Part model, mm, in its own coordinate system. A direction names the side the tool comes from. Round coordinates to 2 decimals unless told otherwise and drop trailing zeros. Order: outer loops, then holes, each group sorted by start corner. A loop starts at its lowest first (then second) coordinate and runs counter-clockwise, first axis right, second up. Notation, with made-up numbers: (-11, 46) -> (40, 46) arc R34 cw to (40, 79) -> close; hole circle Ø4 at (53, 10). An arc over 180 degrees is marked (long way). Return JSON: item names as keys, results as strings. Group by question number.
Autodesk Inventor part; units mm, degrees
ref_plane "YZ Plane" through (0, 0, 0) normal (1, 0, 0) x (0, 1, 0)
ref_plane "XZ Plane" through (0, 0, 0) normal (0, 1, 0) x (-1, 0, 0)
ref_plane "XY Plane" through (0, 0, 0) normal (0, 0, 1) x (1, 0, 0)
sketch "Sketch1" plane through (0, 0, 0) normal (0, 0, 1) x (1, 0, 0)
  circle A0 centre (0, 0) radius 14.75
  circle A1 centre (0, 0) radius 8 construction
  line L0 (-14.75, 0) -> (14.75, 0) construction
  line L1 (-7.5993, -2.5) -> (7.5993, -2.5) construction
  line L2 (-7.5993, 2.5) -> (7.5993, 2.5) construction
  circle A2 centre (0, 0) radius 12.5 construction
  circle A3 centre (0, 0) radius 6.5 construction
  circle A4 centre (0, 0) radius 9.5 construction
  line L3 (0, 0) -> (6.7175, 6.7175) construction
  line L4 (0, -14.75) -> (0, 14.75) construction
  circle A5 centre (0, 0) radius 10.25 construction
  circle A6 centre (0, 10.25) radius 2.75 construction
  circle A7 centre (0, 10.25) radius 3.25 construction
  circle A8 centre (6.7175, 6.7175) radius 2 construction
  circle A9 centre (6.7175, 6.7175) radius 2 construction
  line L5 (-7.6174, -2.525) -> (7.6174, -2.525)
  arc A10 (7.6174, -2.525) -> (7.6174, 2.525) centre (0, 0) ccw
  line L6 (7.6174, 2.525) -> (-7.6174, 2.525)
  arc A11 (-7.6174, 2.525) -> (-7.6174, -2.525) centre (0, 0) ccw
  arc A12 (7.9142, 1.3291) -> (6.3852, 2.525) centre (7.0013, 1.7373) ccw
  arc A13 (6.3852, -2.525) -> (7.9142, -1.3291) centre (7.0013, -1.7373) ccw
  arc A14 (-6.3852, 2.525) -> (-7.9142, 1.3291) centre (-7.0013, 1.7373) ccw
  arc A15 (-7.9142, -1.3291) -> (-6.3852, -2.525) centre (-7.0013, -1.7373) ccw
  circle A16 centre (0, 10.25) radius 1.75 construction
  circle A17 centre (6.7175, 6.7175) radius 3.25 construction
  point P0 (-6.7175, 6.7175)
  point P1 (-6.7175, -6.7175)
  point P2 (6.7175, -6.7175)
  point P3 (-7.9142, 1.3291)
  point P4 (-7.9142, -1.3291)
  point P5 (-6.3852, -2.525)
  point P6 (6.3852, -2.525)
  point P7 (7.9142, -1.3291)
  point P8 (-6.3852, 2.525)
  point P9 (-10.25, 0)
  point P10 (0, -10.25)
  point P11 (10.25, 0)
  dimension "d1" = 16
  dimension "d2" = 5
  dimension "d3" = 25
  dimension "d4" = 29.5
  dimension "d7" = 45
  dimension "d11" = 360
  dimension "d36" = 5.5
  dimension "d37" = 0.5
  dimension "d39" = 4
  dimension "d40" = 0
  dimension "d41" = 0.025
  dimension "d42" = 0.025
  dimension "d43" = 1
  dimension "d47" = 3.5
  dimension "d48" = 0.5
  dimension "d49" = 1
  dimension "d52" = 360
  dimension "d56" = 1
  dimension "d57" = 6.5
extrude "Extrusion1" add sketch "Sketch1" against normal blind 5 contours A0 | A11 L6 A10 L5 | A15 A11 | L5 A15 | L5 A13 | A14 A11 | A10 A13 | A14 L6 | A10 A12 | A12 L6
hole "Hole1" at (0, 0, 0) direction (0, 0, -1) diameter 3.2 end through all
hole "Hole2" [suppressed]
hole "Hole3" at (6.7175, 6.7175, 0) at (-6.7175, 6.7175, 0) at (-6.7175, -6.7175, 0) at (6.7175, -6.7175, 0) direction (0, 0, -1) diameter 4 end through all counterbore diameter 7 counterbore depth 2.5
extrude "Extrusion2" cut sketch "Sketch1" against normal blind 2 contours A11 L6 A10 L5 | A15 A11 | L5 A15 | L5 A13 | A14 A11 | A10 A13 | A14 L6 | A10 A12 | A12 L6
equation "\"d42\" = d41"
properties part number "CrossRollerBearingInnerFlange" material "Aluminum 7075"
(1) Saw through at B-B, the plane y = 5.75. List the corners of the cut face in (x, z), and give its area (3 significant figures).
(2) Probe L1, parallel to X at y = -8.25, z = -1.6; L2, parallel to Y at x = -5, z = -1.1 (3 decimals); L3, parallel to X at y = -4.5, z = -0.95. List the from-to ranges inside material, lowest first. Write a range as [from, to].
(3) Mould opens along X. For faces 1 (the flat face through (-5, 5, -2.5)), 2 (the flat face through (0, -3, -5)), 3 (the cylindrical face through (14.07, 4.43, -2.46)) say: pulls with the +X half, pulls with the -X half, needs draft (parallel to the pull), parting line crosses it, or undercut.
(4) Pin check, flat tips, straight feed: P1, Ø4.5, axis at x = -6.72, y = -6.72, coming from the +Z side; P2, Ø3, axis at y = 3, z = -3, coming from the +X side; P3, Ø3, axis at y = -11.5, z = -0.5, coming from the -X side. Stop position of each tip, or through.
(5) Saw through at C-C, the plane z = -0.9. State how many separate pieces and enclosed holes the cut face has, and give its area (3 significant figures).
(6) Tool access for faces 4 (the flat face through (0, -3, 0)), 5 (the flat face through (2, 0, -2)): list every direction of +Z, -Z, +X, -X, +Y, -Y with a clear straight run to the whole face (end or side of a thin tool).
(7) Saw through at D-D, the plane y = 0. List the corners of the cut face in (x, z), and give its area (3 significant figures).
(8) Saw through at A-A, the plane x = 0. List the corners of the cut face in (y, z) (3 decimals).
Results are:
{
 "1": {"outline": "(-13.58, -5) -> (-8.47, -5) -> (-8.47, -2.5) -> (-10.08, -2.5) -> (-10.08, 0) -> (-13.58, 0) -> close; (-4.97, -5) -> (4.97, -5) -> (4.97, -2.5) -> (3.35, -2.5) -> (3.35, 0) -> (-3.35, 0) -> (-3.35, -2.5) -> (-4.97, -2.5) -> close; (8.47, -5) -> (13.58, -5) -> (13.58, 0) -> (10.08, 0) -> (10.08, -2.5) -> (8.47, -2.5) -> close", "area": "84.7 mm^2"},
 "2": {"L1": "x = [-12.23, -9.86], [-3.57, 3.57], [9.86, 12.23]", "L2": "y = [-13.877, -9.767], [-3.668, -2.525], [2.525, 3.668], [9.767, 13.877]", "L3": "x = [-14.05, -9.43], [-4.01, 4.01], [9.43, 14.05]"},
 "3": {"face 1": "undercut", "face 2": "needs draft", "face 3": "parting line crosses it"},
 "4": {"P1": "stops at z = -2.5", "P2": "stops at x = 14.67", "P3": "stops at x = -10.84"},
 "5": {"separate pieces": "1", "enclosed holes": "5", "area": "449 mm^2"},
 "6": {"face 4": "+Z, +X, -X, +Y, -Y", "face 5": "+Z"},
 "7": {"outline": "(-14.75, -5) -> (-1.6, -5) -> (-1.6, -2) -> (-8.02, -2) -> (-8.02, 0) -> (-14.75, 0) -> close; (1.6, -5) -> (14.75, -5) -> (14.75, 0) -> (8.02, 0) -> (8.02, -2) -> (1.6, -2) -> close", "area": "106 mm^2"},
 "8": {"outline": "(-14.75, -5) -> (-1.6, -5) -> (-1.6, -2) -> (-2.525, -2) -> (-2.525, 0) -> (-14.75, 0) -> close; (1.6, -5) -> (14.75, -5) -> (14.75, 0) -> (2.525, 0) -> (2.525, -2) -> (1.6, -2) -> close"}
}
